Model file for the job. Use its own axes, mm. A direction names the side the tool comes from. Round coordinates to 2 decimals unless told otherwise and drop trailing zeros. Write each loop counter-clockwise with the first axis right and the second up, starting at its lowest first coordinate (ties: lowest second). Pieces come first, ordered by that corner, then holes. Notation, with made-up numbers: (-4.75, -29.75) - (5.25, -29.75) arc R12 cw to (5.25, -21.75) - close; hole circle Ø5 at (71.5, 64.25). An arc over 180 degrees is marked (long way). One line per item, written item: value.
from build123d import *

# Parameters (mm, degrees)
SKETCH_1_W          = 30
SKETCH_1_H          = 3
EXTRUDE_1_DEPTH     = 3
SKETCH_2_R          = 1.75
CUT_EXTRUDE_1_DEPTH = 10
SKETCH_3_R          = 1.75
CUT_EXTRUDE_2_DEPTH = 10
CHAMFER_1_SIZE      = 2
CHAMFER_2_SIZE      = 2
CUT_EXTRUDE_3_DEPTH = 3


with BuildPart() as part:
    # Эскиз1 → Бобышка-Вытянуть1 (new body)
    with BuildSketch(Plane.XY):
        Polygon((-27.5, 50), (-27.5, -50), (27.5, -50), (27.5, 50), (15, 50), (15, 47), (-15, 47), (-15, 50), align=None)
        with Locations((0, 48.5)):
            Rectangle(SKETCH_1_W, SKETCH_1_H)
        with Locations((0, 51.5)):
            Rectangle(SKETCH_1_W, SKETCH_1_H)
    extrude(amount=EXTRUDE_1_DEPTH)

    # Эскиз2 → Вырез-Вытянуть1 (cut)
    with BuildSketch(Plane.XY.offset(3)):
        with Locations((-15.35, 39.7)):
            Circle(SKETCH_2_R)
        with Locations((15.35, 39.7)):
            Circle(SKETCH_2_R)
        with Locations((15.35, 9)):
            Circle(SKETCH_2_R)
        with Locations((-15.35, 9)):
            Circle(SKETCH_2_R)
        with Locations((-15.35, -9)):
            Circle(SKETCH_2_R)
        with Locations((15.35, -9)):
            Circle(SKETCH_2_R)
        with Locations((15.35, -39.7)):
            Circle(SKETCH_2_R)
        with Locations((-15.35, -39.7)):
            Circle(SKETCH_2_R)
    extrude(amount=-CUT_EXTRUDE_1_DEPTH, mode=Mode.SUBTRACT)

    # Эскиз3 → Вырез-Вытянуть2 (cut)
    with BuildSketch(Plane(origin=(0, 0, 0), x_dir=(-1, 0, 0), z_dir=(0, 0, -1))):
        with Locations((-22.5, 24.35)):
            Circle(SKETCH_3_R)
        with Locations((-12.5, 24.35)):
            Circle(SKETCH_3_R)
        with Locations((-5, 24.35)):
            Circle(SKETCH_3_R)
        with Locations((5, 24.35)):
            Circle(SKETCH_3_R)
        with Locations((12.5, 24.35)):
            Circle(SKETCH_3_R)
        with Locations((22.5, 24.35)):
            Circle(SKETCH_3_R)
        with Locations(Location((22.5, -24.35, 0), (0, 0, 180))):
            Circle(SKETCH_3_R)
        with Locations(Location((12.5, -24.35, 0), (0, 0, 180))):
            Circle(SKETCH_3_R)
        with Locations(Location((5, -24.35, 0), (0, 0, 180))):
            Circle(SKETCH_3_R)
        with Locations(Location((-5, -24.35, 0), (0, 0, 180))):
            Circle(SKETCH_3_R)
        with Locations(Location((-12.5, -24.35, 0), (0, 0, 180))):
            Circle(SKETCH_3_R)
        with Locations(Location((-22.5, -24.35, 0), (0, 0, 180))):
            Circle(SKETCH_3_R)
    extrude(amount=-CUT_EXTRUDE_2_DEPTH, mode=Mode.SUBTRACT)

    # Фаска1
    chamfer_1_edges = [part.edges().sort_by_distance(p)[0] for p in [
        (-17.1, -9, 0),
        (-17.1, 9, 0),
        (13.6, 9, 0),
        (-17.1, 39.7, 0),
        (13.6, -9, 0),
        (13.6, -39.7, 0),
        (-17.1, -39.7, 0),
        (13.6, 39.7, 0),
    ]]
    chamfer(chamfer_1_edges, length=CHAMFER_1_SIZE)

    # Фаска2
    chamfer_2_edges = [part.edges().sort_by_distance(p)[0] for p in [
        (14.25, 24.35, 3),
        (3.25, -24.35, 3),
        (10.75, -24.35, 3),
        (20.75, -24.35, 3),
        (24.25, 24.35, 3),
        (-6.75, -24.35, 3),
        (-14.25, -24.35, 3),
        (-24.25, -24.35, 3),
        (-20.75, 24.35, 3),
        (-10.75, 24.35, 3),
        (-3.25, 24.35, 3),
        (6.75, 24.35, 3),
    ]]
    chamfer(chamfer_2_edges, length=CHAMFER_2_SIZE - 0.0001)  # a hair under: the kernel refuses the full size

    # Эскиз4 → Вырез-Вытянуть3 (cut)
    with BuildSketch(Plane(origin=(0, 0, 0), x_dir=(-1, 0, 0), z_dir=(0, 0, -1))):
        with BuildLine():
            Line((-11.5, 5), (11.5, 5))
            ThreePointArc((11.5, 5), (16.5, 0), (11.5, -5))
            Line((11.5, -5), (-11.5, -5))
            ThreePointArc((-11.5, -5), (-16.5, 0), (-11.5, 5))
        make_face()
    extrude(amount=-CUT_EXTRUDE_3_DEPTH, mode=Mode.SUBTRACT)


solid = part.part
1. Drop flat-ended pins along their axis: pin 1 (3 mm diameter, centred on x = -15.35, y = 9, fed in from -Z); pin 2 (1.5 mm diameter, centred on x = -19, z = 1.5, fed in from +Y); pin 3 (4.5 mm diameter, centred on x = 15.35, y = 9, fed in from +Z); pin 4 (5.5 mm diameter, centred on x = 12.5, y = 24.35, fed in from +Z). Give the stop position or say it passes through.
Report:
pin 1: through
pin 2: y = 50
pin 3: z = 3
pin 4: z = 2
2. Mould opens along Y. For faces 1 (the face through (0, -9, 0)), 2 (the face through (-21, 50, 1)), 3 (the face through (-4.19, -22.8, 0.49)) say: released by +Y, released by -Y, zero draft, split by the parting line, or undercut.
Report:
face 1: zero draft
face 2: released by +Y
face 3: undercut
3. Band-saw the part on B-B on x = -5. Write the cut outline in (y, z).
Report:
outline: (-50, 0) - (-26.1, 0) - (-26.1, 1) - (-28.1, 3) - (-50, 3) - close; (-22.6, 0) - (-5, 0) - (-5, 3) - (-20.6, 3) - (-22.6, 1) - close; (5, 0) - (22.6, 0) - (22.6, 1) - (20.6, 3) - (5, 3) - close; (26.1, 0) - (53, 0) - (53, 3) - (28.1, 3) - (26.1, 1) - close
4. Wall check: probe 1 along Y at (x, z) = (5, 0.6); probe 2 along Y at (x, z) = (-22.5, 0.55); probe 3 along Y at (x, z) = (10.5, 2.25). Give the ranges that are in metal, low to high. Write a range as [from, to].
Report:
probe 1: [-50, -26.1], [-22.6, -5], [5, 22.6], [26.1, 53]
probe 2: [-50, -26.1], [-22.6, 22.6], [26.1, 50]
probe 3: [-50, -26.59], [-22.11, -5], [5, 22.11], [26.59, 53]
5. Band-saw the part on A-A on y = -9. Write the cut outline in (x, z).
Report:
outline: (-27.5, 0) - (-19.1, 0) - (-17.1, 2) - (-17.1, 3) - (-27.5, 3) - close; (-13.6, 2) - (-11.6, 0) - (11.6, 0) - (13.6, 2) - (13.6, 3) - (-13.6, 3) - close; (17.1, 2) - (19.1, 0) - (27.5, 0) - (27.5, 3) - (17.1, 3) - close
6. Tool access for faces 4 (the face through (-15, 51, 1)), 5 (the face through (27.5, -1, 1)), 6 (the face through (15, 51, 1)): list every direction of +Z, -Z, +X, -X, +Y, -Y with a clear straight run to the whole face (end or side of a thin tool).
Report:
face 4: +Z, -Z, -X, +Y
face 5: +Z, -Z, +X, +Y, -Y
face 6: +Z, -Z, +X, +Y
7. Band-saw the part on C-C on z = 0.55. State how many separate pieces and enclosed holes the cut face has, plus the area to 3 significant figures.
Report:
separate pieces: 1
enclosed holes: 21
area: 4,910 mm²
